The listing builds one solid part. Answer for the finished solid, in the listing's coordinates (mm). Coordinates: 2 decimals unless noted, no trailing zeros. Order: outer loops, then holes, each group sorted by start corner. A loop starts at its lowest first (then second) coordinate and runs counter-clockwise, first axis right, second up. Notation, with made-up numbers: (17.25, 1.25) - (45.25, 1.25) arc R14 ccw to (45.25, 21.25) - close; hole circle Ø3 at (-10.5, 30.25). An arc over 180 degrees is marked (long way). Use a Markdown table: item, result. Add a question column.
Item 1: The mould has two halves that part along Z. Classify faces 1 (the flat face through (-15, 0, -45)), 2 (the cylindrical face through (-48.454, 23.664, -15.259)), 3 (the cylindrical face through (-43.876, 25.157, -13.817)): released by +Z, released by -Z, zero draft, split by the parting line, or undercut.
Item 2: The part is cut by section A-A, the plane x = 0. Give the vertices of the cut face in (y, z).
Item 3: The part is cut by section B-B, the plane z = 0. Give the vertices of the cut face in (x, y), then the cut area to 3 significant figures.
Item 4: Find the intervals of material crossed by line 1 along Z through (x, y) = (0, 12); line 2 along Y through (x, z) = (-48.05, 0); line 3 along X through (y, z) = (30, 42), in increasing order.
Item 5: Flat-ended cylindrical pins translate along their axes: P1, Ø1.5, axis at y = 18.5, z = 31.5, coming from the +X side; P2, Ø12, axis at y = 39, z = 11.5, coming from the +X side; P3, Ø8, axis at x = 15, z = 37, coming from the +Y side; P4, Ø8, axis at y = 28, z = 28.5, coming from the +X side. Find the tip coordinate at first contact, or state that the pin passes through.
Item 6: The part is cut by section D-D, the plane y = 4.5. Give the vertices of the cut face in (x, z).
Autodesk Inventor part; units mm, degrees
ref_plane "YZ Plane" through (0, 0, 0) normal (1, 0, 0) x (0, 1, 0)
ref_plane "XZ Plane" through (0, 0, 0) normal (0, 1, 0) x (-1, 0, 0)
ref_plane "XY Plane" through (0, 0, 0) normal (0, 0, 1) x (1, 0, 0)
sketch "Sketch1" plane through (0, 0, 0) normal (0, 1, 0) x (-1, 0, 0)
  circle A0 centre (0, 0) radius 46
  circle A1 centre (0, 0) radius 50.8
  dimension "d0" = 92
  dimension "d1" = 101.6
extrude "Extrusion1" add sketch "Sketch1" along normal blind 50
chamfer "Chamfer1" distance 2 angle 45 1 edges at (50.8, 50, 0)
chamfer "Chamfer2" distance 1 angle 45 1 edges at (46, 0, 0)
sketch "Sketch2" plane through (0, 0, 0) normal (1, 0, 0) x (0, 1, 0)
  circle A0 centre (30, 0) radius 2.5
  line L0 (50, 46) -> (50, -46)
  point P0 (0, 0)
  dimension "d10" = 5
  dimension "d11" = 20
extrude "Extrusion2" cut sketch "Sketch2" along normal through all both and the other way through all
properties part number "HubSparHole90"
Solution:
| question | item | result |
|---|---|---|
| 1 | face 1 | zero draft |
| 1 | face 2 | split by the parting line |
| 1 | face 3 | undercut |
| 2 | outline | (0, -50.8) - (48, -50.8) - (50, -48.8) - (50, -46) - (1, -46) - (0, -47) - close; (0, 47) - (1, 46) - (50, 46) - (50, 48.8) - (48, 50.8) - (0, 50.8) - close |
| 3 | outline | (-50.8, 0) - (-47, 0) - (-46, 1) - (-46, 27.5) - (-50.8, 27.5) - close; (-50.8, 32.5) - (-46, 32.5) - (-46, 50) - (-48.8, 50) - (-50.8, 48) - close; (46, 1) - (47, 0) - (50.8, 0) - (50.8, 27.5) - (46, 27.5) - close; (46, 32.5) - (50.8, 32.5) - (50.8, 48) - (48.8, 50) - (46, 50) - close |
| 3 | area | 427 mm2 |
| 4 | line 1 | z = -50.8 to -46, 46 to 50.8 |
| 4 | line 2 | y = 0 to 27.5, 32.5 to 50 |
| 4 | line 3 | x = -28.58 to -18.76, 18.76 to 28.58 |
| 5 | P1 | stops at x = 40.44 |
| 5 | P2 | stops at x = 50.5 |
| 5 | P3 | passes through |
| 5 | P4 | stops at x = 44.5 |
| 6 | outline | circle Ø101.6 at (0, 0); hole circle Ø92 at (0, 0) |
